```python
from build123d import *

# Parameters (mm, degrees)
CROQUIS2_R              = 35
SALIENTE_EXTRUIR1_DEPTH = 3.5
CROQUIS6_R              = 3
CORTAR_EXTRUIR2_DEPTH   = 2
CROQUIS7_R              = 1.5
CORTAR_EXTRUIR3_DEPTH   = 50.621064076
CROQUIS9_R              = 1.25
CORTAR_EXTRUIR5_DEPTH   = 50.621064076
CROQUIS10_W             = 9.2
CROQUIS10_H             = 20.3
CORTAR_EXTRUIR6_DEPTH   = 10


with BuildPart() as part:
    # Croquis2 → Saliente-Extruir1 (new body)
    with BuildSketch(Plane.XY):
        Circle(CROQUIS2_R)
    extrude(amount=SALIENTE_EXTRUIR1_DEPTH)

    # Croquis6 → Cortar-Extruir2 (cut)
    with BuildSketch(Plane.XY.offset(3.5)):
        with Locations((0, 26.5)):
            Circle(CROQUIS6_R)
        with Locations((22.9496732, -13.25)):
            Circle(CROQUIS6_R)
        with Locations((-22.9496732, -13.25)):
            Circle(CROQUIS6_R)
    extrude(amount=-CORTAR_EXTRUIR2_DEPTH, mode=Mode.SUBTRACT)

    # Croquis7 → Cortar-Extruir3 (cut, through all)
    with BuildSketch(Plane.XY.offset(3.5)):
        with Locations((0, 26.5)):
            Circle(CROQUIS7_R)
        with Locations((22.9496732, -13.25)):
            Circle(CROQUIS7_R)
        with Locations((-22.9496732, -13.25)):
            Circle(CROQUIS7_R)
    extrude(amount=-CORTAR_EXTRUIR3_DEPTH, mode=Mode.SUBTRACT)

    # Croquis9 → Cortar-Extruir5 (cut, through all)
    with BuildSketch(Plane(origin=(0, 0, 0), x_dir=(-1, 0, 0), z_dir=(0, 0, -1))):
        with Locations((-24, 1.3)):
            Circle(CROQUIS9_R)
        with Locations((11, 1.3)):
            Circle(CROQUIS9_R)
        with Locations((29.5, 1.3)):
            Circle(CROQUIS9_R)
    extrude(amount=-CORTAR_EXTRUIR5_DEPTH, mode=Mode.SUBTRACT)

    # Croquis10 → Cortar-Extruir6 (cut)
    with BuildSketch(Plane(origin=(0, 0, 0), x_dir=(-1, 0, 0), z_dir=(0, 0, -1))):
        with Locations((20.25, 5)):
            Rectangle(CROQUIS10_W, CROQUIS10_H)
    extrude(amount=-CORTAR_EXTRUIR6_DEPTH, mode=Mode.SUBTRACT)


solid = part.part
```
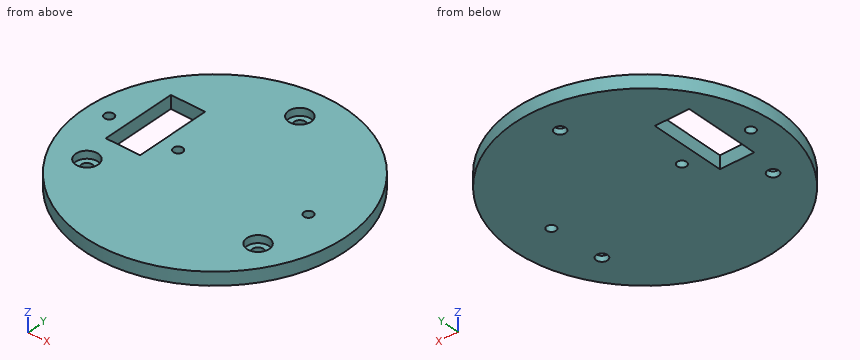
Source: CAD feature listing. Evaluate the final solid. Frame: model axes, mm. Coordinates: 2 decimals unless noted, no trailing zeros. Loops run counter-clockwise (first coordinate to the right, second up) from the corner with the lowest first, then second, coordinate; pieces in that order, holes last. Notation, with made-up numbers: M 57.5,44.5 L 70.5,44.5 A17 ccw 70.5,64.5 Z; hole C -36.75,73.25 d3. An arc over 180 degrees is marked long. Use CSV: the item, a comma, the result in double quotes.
(1) Cut plane B-B on x = 0. Return loops of the section in (y, z), and give its area (4 significant figures).
Answers follow:
outline,"M -35,0 L 25,0 L 25,1.5 L 23.5,1.5 L 23.5,3.5 L -35,3.5 Z; M 28,0 L 35,0 L 35,3.5 L 29.5,3.5 L 29.5,1.5 L 28,1.5 Z"
area,"228.5 mm²"
(2) Contact query for flat-ended pins moving along their axis: pin 1 (1.8 mm diameter, centred on x = 0, y = 26.5, fed in from -Z); pin 2 (3.5 mm diameter, centred on x = -22.95, y = -13.25, fed in from +Z); pin 3 (1 mm diameter, centred on x = -20, z = 2.5, fed in from -Y). Output: stop coordinate, or through.
Answers follow:
pin 1,"through"
pin 2,"z = 1.5"
pin 3,"y = -29.06"
(3) Cut plane D-D on x = -22.5. Return loops of the section in (y, z).
Answers follow:
outline,"M -26.81,0 L -14.68,0 L -14.68,1.5 L -16.22,1.5 L -16.22,3.5 L -26.81,3.5 Z; M -11.82,0 L -5.15,0 L -5.15,3.5 L -10.28,3.5 L -10.28,1.5 L -11.82,1.5 Z; M 15.15,0 L 26.81,0 L 26.81,3.5 L 15.15,3.5 Z"
(4) Cut plane C-C on y = 26.5. Return loops of the section in (x, z).
Answers follow:
outline,"M -22.86,0 L -1.5,0 L -1.5,1.5 L -3,1.5 L -3,3.5 L -22.86,3.5 Z; M 1.5,0 L 22.86,0 L 22.86,3.5 L 3,3.5 L 3,1.5 L 1.5,1.5 Z"
(5) Line query: line 1 (X direction, y = -13, z = 2.55); line 2 (Y direction, x = -23.5, z = 2.3); line 3 (Y direction, x = 0, z = 2.1). Output: solid intervals per line, ascending. Write a range as [from, to].
Answers follow:
line 1,"[-32.5, -25.94], [-19.96, 19.96], [25.94, 32.5]"
line 2,"[-25.94, -16.2], [-10.3, -5.15], [15.15, 25.94]"
line 3,"[-35, 23.5], [29.5, 35]"
(6) Cut plane A-A on z = 2.3. Return loops of the section in (x, y).
Answers follow:
outline,"C 0,0 d70; hole C -29.5,1.3 d2.5; hole C -22.95,-13.25 d6; hole M -24.85,-5.15 L -15.65,-5.15 L -15.65,15.15 L -24.85,15.15 Z; hole C -11,1.3 d2.5; hole C 0,26.5 d6; hole C 22.95,-13.25 d6; hole C 24,1.3 d2.5"
